Can you work these out from the drawing? Everything is in mm from the part's minimum corner. Round coordinates to 2 decimals unless told otherwise and drop trailing zeros. Write each loop counter-clockwise with the first axis right and the second up, starting at its lowest first coordinate (ties: lowest second). Pieces come first, ordered by that corner, then holes. Notation, with made-up numbers: (-19.75, 76) -> (-4.75, 76) arc R12 ccw to (-4.75, 92) -> close; hole circle Ø4 at (-24.75, 32). An arc over 180 degrees is marked (long way). Put each result on its own line as item: value. Start each with the question number.
1. Suppose I cut it at A-A (x = 12.5). Please give me the cut outline in (y, z).
2. Suppose I cut it at B-B (z = 7.5). Please give me the cut outline in (x, y), then the cut area to 3 significant figures.
3. Suppose I cut it at C-C (y = 12). Please give me the cut outline in (x, z).
4. For pin 1 (8 mm diameter, centred on x = 16.5, z = 5.5, fed in from -Y), with a flat end and sliding along its axis, tell me the tip position at first contact or that it passes through.
5. We'd pull the mould along X, two halves only. Please class the marked faces 1, 2, 3 and 4: +X half, -X half, draft (parallel to the pull), parting line (faces both ways), or undercut.
6. Suppose I cut it at D-D (y = 1.5). Please give me the cut outline in (x, z).
7. I need wall thicknesses on probe 1 along X at (y, z) = (18.75, 9); probe 2 along X at (y, z) = (4.75, 13.25); probe 3 along Y at (x, z) = (26, 13). Which ranges of each line are inside material? Lowest first, please. Write a range as from..to.
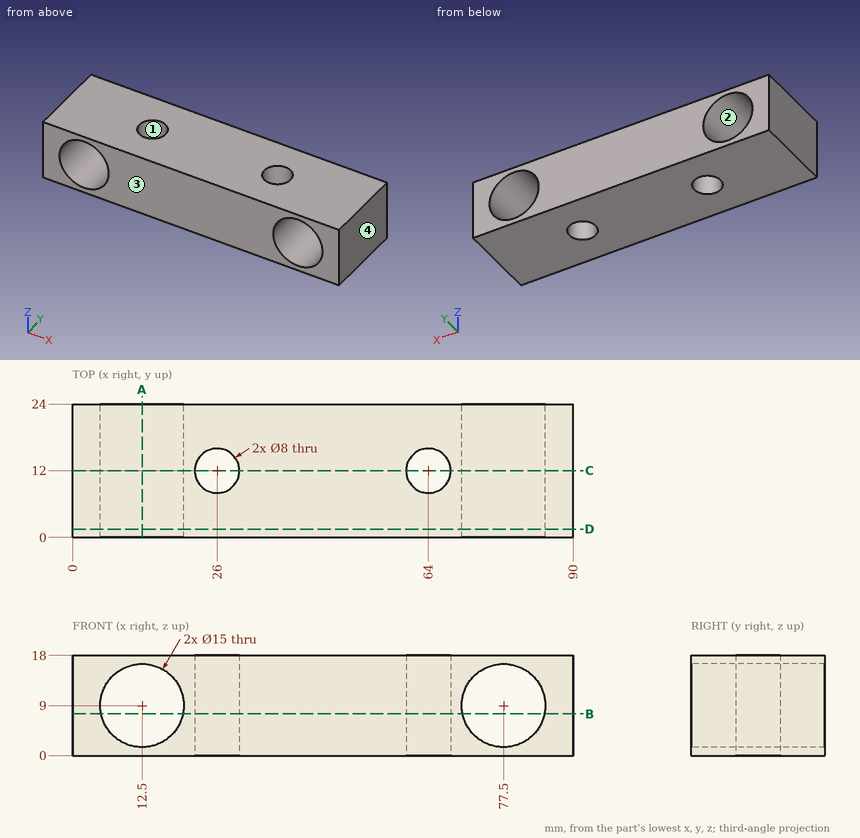
Verdict:
1. outline: (0, 0) -> (24, 0) -> (24, 1.5) -> (0, 1.5) -> close; (0, 16.5) -> (24, 16.5) -> (24, 18) -> (0, 18) -> close
2. outline: (0, 0) -> (5.15, 0) -> (5.15, 24) -> (0, 24) -> close; (19.85, 0) -> (70.15, 0) -> (70.15, 24) -> (19.85, 24) -> close; (84.85, 0) -> (90, 0) -> (90, 24) -> (84.85, 24) -> close; hole circle Ø8 at (26, 12); hole circle Ø8 at (64, 12)
2. area: 1,350 mm^2
3. outline: (0, 0) -> (22, 0) -> (22, 18) -> (0, 18) -> close; (30, 0) -> (60, 0) -> (60, 18) -> (30, 18) -> close; (68, 0) -> (90, 0) -> (90, 18) -> (68, 18) -> close; hole circle Ø15 at (12.5, 9); hole circle Ø15 at (77.5, 9)
4. pin 1: stops at y = 0
5. face 1: undercut
5. face 2: undercut
5. face 3: draft
5. face 4: +X half
6. outline: (0, 0) -> (90, 0) -> (90, 18) -> (0, 18) -> close; hole circle Ø15 at (12.5, 9); hole circle Ø15 at (77.5, 9)
7. probe 1: x = 0..5, 20..70, 85..90
7. probe 2: x = 0..6.32, 18.68..71.32, 83.68..90
7. probe 3: y = 0..8, 16..24
